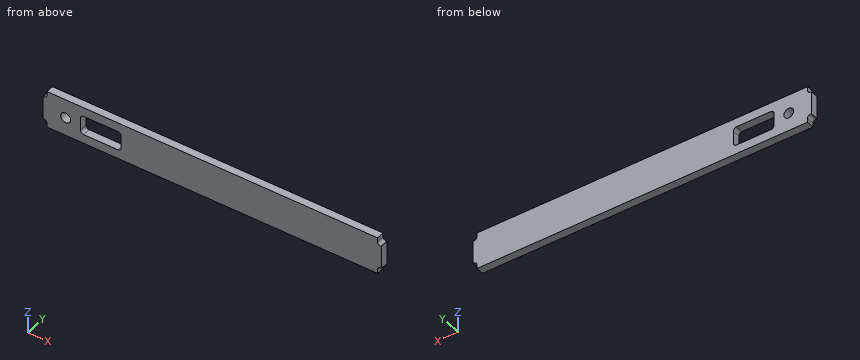
from build123d import *

# Parameters (mm, degrees)
SKETCH1_W               = 673.1
SKETCH1_H               = 74.742799968
BOSS_EXTRUDE1_DEPTH     = 15.875
SKETCH3_R               = 10.1
CUT_EXTRUDE1_DEPTH      = 1
CUT_EXTRUDE1_DEPTH_BACK = 16.875
SKETCH4_W               = 7.9375
SKETCH4_H               = 46.167799968
BOSS_EXTRUDE3_DEPTH     = 15.875
FILLET2_R               = 6.35
SKETCH5_W               = 82.804
SKETCH5_H               = 38.354
CUT_EXTRUDE2_DEPTH      = 1
CUT_EXTRUDE2_DEPTH_BACK = 16.875
FILLET3_R               = 6.35


with BuildPart() as part:
    # Sketch1 → Boss-Extrude1 (new body)
    with BuildSketch(Plane(origin=(0, 0, 0), x_dir=(1, 0, 0), z_dir=(0, 1, 0))):
        Rectangle(SKETCH1_W, SKETCH1_H)
    extrude(amount=BOSS_EXTRUDE1_DEPTH)

    # Sketch3 → Cut-Extrude1 (cut, two sides)
    with BuildSketch(Plane(origin=(0, 15.875, 0), x_dir=(1, 0, 0), z_dir=(0, 1, 0))) as cut_extrude1_sk:
        with Locations((-298.45, 0.728600016)):
            Circle(SKETCH3_R)
    extrude(amount=CUT_EXTRUDE1_DEPTH, mode=Mode.SUBTRACT)
    extrude(cut_extrude1_sk.sketch, amount=-CUT_EXTRUDE1_DEPTH_BACK, mode=Mode.SUBTRACT)

    # Sketch4 → Boss-Extrude3 (add)
    with BuildSketch(Plane(origin=(0, 15.875, 0), x_dir=(1, 0, 0), z_dir=(0, 1, 0))):
        with Locations((-340.51875, 0)):
            Rectangle(SKETCH4_W, SKETCH4_H)
        with Locations((340.51875, 0)):
            Rectangle(SKETCH4_W, SKETCH4_H)
    extrude(amount=-BOSS_EXTRUDE3_DEPTH)

    # Fillet2
    fillet2_edges = [part.edges().sort_by_distance(p)[0] for p in [
        (-336.55, 7.9375, 23.083899984),
        (-336.55, 7.9375, -23.083899984),
        (336.55, 7.9375, 23.083899984),
        (336.55, 7.9375, -23.083899984),
    ]]
    fillet(fillet2_edges, radius=FILLET2_R)

    # Sketch5 → Cut-Extrude2 (cut, two sides)
    with BuildSketch(Plane(origin=(0, 15.875, 0), x_dir=(1, 0, 0), z_dir=(0, 1, 0))) as cut_extrude2_sk:
        with Locations((-226.8855, 0)):
            Rectangle(SKETCH5_W, SKETCH5_H)
    extrude(amount=CUT_EXTRUDE2_DEPTH, mode=Mode.SUBTRACT)
    extrude(cut_extrude2_sk.sketch, amount=-CUT_EXTRUDE2_DEPTH_BACK, mode=Mode.SUBTRACT)

    # Fillet3
    fillet3_edges = [part.edges().sort_by_distance(p)[0] for p in [
        (-268.2875, 7.9375, 19.177),
        (-268.2875, 7.9375, -19.177),
        (-185.4835, 7.9375, -19.177),
        (-185.4835, 7.9375, 19.177),
    ]]
    fillet(fillet3_edges, radius=FILLET3_R)


solid = part.part
Check sheet for the modelled part. Datum: model origin and axes. Units: mm. Give positions to 0.01 mm unless a question says otherwise; leave off trailing zeros. Loops run counter-clockwise (first coordinate to the right, second up) from the corner with the lowest first, then second, coordinate; pieces in that order, holes last. Notation, with made-up numbers: M 10.25,-27 L 66.25,-27 A18 cw 66.25,2 Z; hole C 49,15 d4. An arc over 180 degrees is marked long. Answer as a JSON object with one key per item and string values. Group by question number.
Q1. Go/stop test with flat-tipped pins: P1, Ø4, axis at y = 5, z = -35, coming from the -X side; P2, Ø1.7, axis at x = 344, y = 9, coming from the -Z side; P3, Ø6.5, axis at y = 5, z = 35, coming from the +X side. Record where each tip stops, or that it passes through.
Q2. Material ranges on line 1 along Z through (x, y) = (-298.45, 12.5); line 2 along Z through (x, y) = (-242, 13.75); line 3 along X through (y, z) = (7.75, 4), recorded low to high. Write a range as [from, to].
Q3. Cross-section at A-A on x = -298.45. Record the cut outline in (y, z) (3 decimals).
Q4. Cross-section at B-B on y = 7.75. Record the cut outline in (x, z), then the cut area to 3 significant figures.
Evaluation:
{
 "1": {"P1": "stops at x = -336.55", "P2": "stops at z = -23.08", "P3": "stops at x = 336.55"},
 "2": {"line 1": "z = [-37.37, -10.83], [9.37, 37.37]", "line 2": "z = [-37.37, -19.18], [19.18, 37.37]", "line 3": "x = [-344.49, -307.37], [-289.53, -268.29], [-185.48, 344.49]"},
 "3": {"outline": "M 0,-37.371 L 15.875,-37.371 L 15.875,-10.829 L 0,-10.829 Z; M 0,9.371 L 15.875,9.371 L 15.875,37.371 L 0,37.371 Z"},
 "4": {"outline": "M -344.49,-23.08 L -342.9,-23.08 A6.35 cw -336.55,-29.43 L -336.55,-37.37 L 336.55,-37.37 L 336.55,-29.43 A6.35 cw 342.9,-23.08 L 344.49,-23.08 L 344.49,23.08 L 342.9,23.08 A6.35 cw 336.55,29.43 L 336.55,37.37 L -336.55,37.37 L -336.55,29.43 A6.35 cw -342.9,23.08 L -344.49,23.08 Z; hole C -298.45,-0.73 d20.2; hole M -268.29,-12.83 A6.35 ccw -261.94,-19.18 L -191.83,-19.18 A6.35 ccw -185.48,-12.83 L -185.48,12.83 A6.35 ccw -191.83,19.18 L -261.94,19.18 A6.35 ccw -268.29,12.83 Z", "area": "47,600 mm2"}
}
